Source: three-view drawing plus pictorial views. Frame: mm from the lowest corner of the part. A direction names the side the tool comes from. Coordinates: 2 decimals unless noted, no trailing zeros. Loops run counter-clockwise (first coordinate to the right, second up) from the corner with the lowest first, then second, coordinate; pieces in that order, holes last. Notation, with made-up numbers: M 34,-35 L 63,-35 A25 ccw 63,-10 Z; hole C 23.25,40 d10. An arc over 180 degrees is marked long. Write each question's results on one line, items separated by ' | '. Start each with the question number.
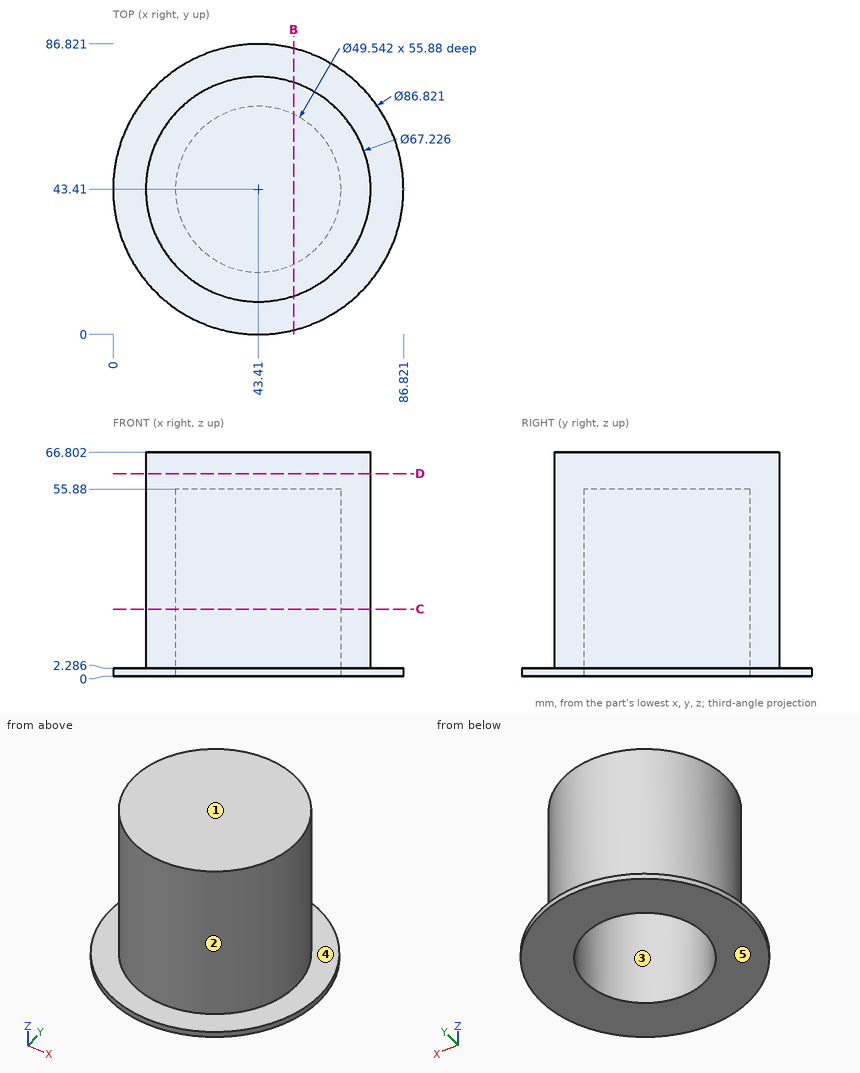
Item 1: Section B-B, the plane x = 54. Return loops of the section in (y, z) (1 decimal), plus the area to 3 significant figures.
Item 2: Section D-D, the plane z = 60.5. Return loops of the section in (x, y).
Item 3: Ray query, L1, parallel to Z at x = 51, y = 81; L2, parallel to Z at x = 51, y = 25.5; L3, parallel to X at y = 58, z = 20.5. Return the intervals inside material, ascending. Write a range as [from, to].
Item 4: Pull-direction query (X, two-part tool) for the marked faces 1, 2 and 3; classes: released by +X, released by -X, zero draft, split by the parting line, or undercut.
Item 5: Set-up query: the marked faces 4 and 5. Return all of +Z, -Z, +X, -X, +Y, -Y with unobstructed straight access to the full face (end or side cutting, diameter ignored); none if empty.
Item 6: Section C-C, the plane z = 20. Return loops of the section in (x, y).
Item 7: Contact query for flat-ended pins moving along their axis: P1, Ø1, axis at y = 68.5, z = 7, coming from the +X side; P2, Ø8, axis at x = 72.5, z = 51.5, coming from the +Y side; P3, Ø4, axis at x = 59, y = 75, coming from the -Z side; P4, Ø3, axis at x = 30, z = 57, coming from the +Y side. Output: stop coordinate, or through.
Solutions:
1) outline: M 1.3,0 L 21,0 L 21,55.9 L 65.8,55.9 L 65.8,0 L 85.5,0 L 85.5,2.3 L 75.3,2.3 L 75.3,66.8 L 11.5,66.8 L 11.5,2.3 L 1.3,2.3 Z | area: 1,810 mm²
2) outline: C 43.41,43.41 d67.23
3) L1: z = [0, 2.29] | L2: z = [55.88, 66.8] | L3: x = [13.13, 23.39], [63.43, 73.69]
4) face 1: zero draft | face 2: split by the parting line | face 3: undercut
5) face 4: +Z | face 5: -Z, +X, -X, +Y, -Y
6) outline: C 43.41,43.41 d67.23; hole C 43.41,43.41 d49.54
7) P1: stops at x = 66.33 | P2: stops at y = 65.78 | P3: stops at z = 0 | P4: stops at y = 74.84
